Could you check a few things on this drawing? It's one solid part, dimensions in mm from its lowest x, y, z. Round coordinates to 2 decimals unless told otherwise and drop trailing zeros. Write each loop counter-clockwise with the first axis right and the second up, starting at its lowest first coordinate (ties: lowest second). Pieces come first, ordered by that corner, then holes. Notation, with made-up numbers: (51, 52.25) - (71, 52.25) arc R16 ccw to (71, 56.25) - close; hole circle Ø5 at (86, 10). An arc over 180 degrees is marked (long way). Put each result on its own line as item: value.
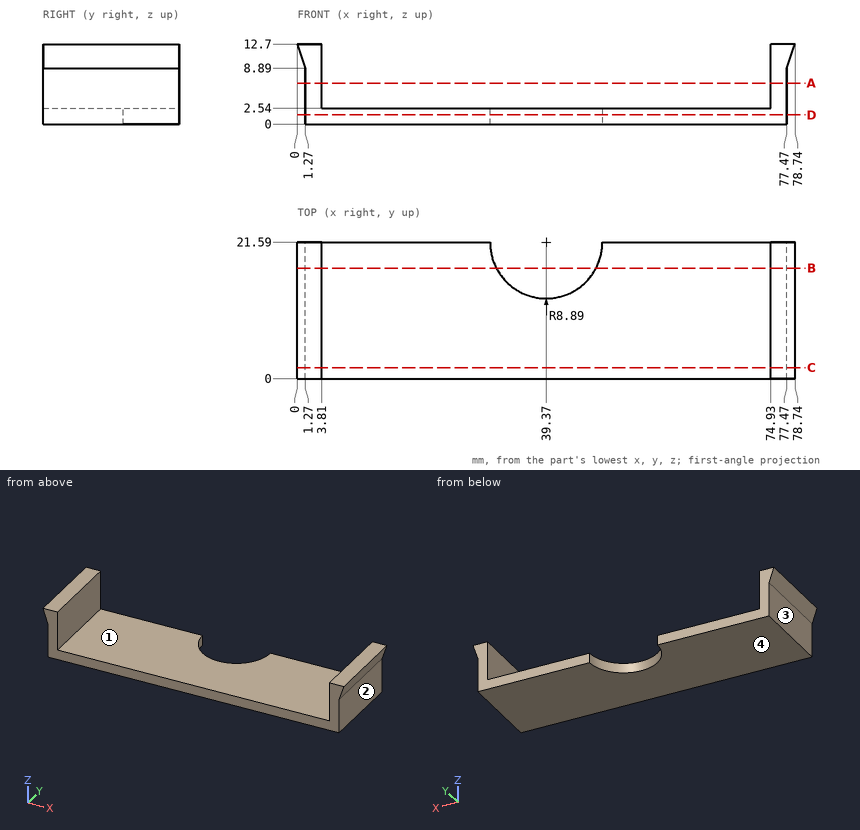
(1) Please list where these lines run through material, in increasing order: probe 1 along X at (y, z) = (20.5, 4.75); probe 2 along Z at (x, y) = (43, 10.5); probe 3 along X at (y, z) = (1, 1). Write a range as from..to.
Values found:
probe 1: x = 1.27..3.81, 74.93..77.47
probe 2: z = 0..2.54
probe 3: x = 1.27..77.47
(2) Imagine slicing it at D-D, the plane z = 1.5. List the corners of the cut face in (x, y) for me.
Values found:
outline: (1.27, 0) - (77.47, 0) - (77.47, 21.59) - (48.26, 21.59) arc R8.89 cw to (30.48, 21.59) - (1.27, 21.59) - close
(3) Imagine slicing it at C-C, the plane y = 1.75. List the corners of the cut face in (x, z) for me, then the cut area to 3 significant figures.
Values found:
outline: (0, 12.7) - (1.27, 8.89) - (1.27, 0) - (77.47, 0) - (77.47, 8.89) - (78.74, 12.7) - (74.93, 12.7) - (74.93, 2.54) - (3.81, 2.54) - (3.81, 12.7) - close
area: 250 mm^2
(4) If we mould it in two halves opening along X, with no side actions, what happens to the marked faces 1, 2, 3 and 4? For each: pulls with the +X half, pulls with the -X half, needs draft (parallel to the pull), parting line crosses it, or undercut.
Values found:
face 1: undercut
face 2: pulls with the +X half
face 3: pulls with the -X half
face 4: needs draft
(5) Imagine slicing it at B-B, the plane y = 17.5. List the corners of the cut face in (x, z) for me, then the cut area to 3 significant figures.
Values found:
outline: (0, 12.7) - (1.27, 8.89) - (1.27, 0) - (31.48, 0) - (31.48, 2.54) - (3.81, 2.54) - (3.81, 12.7) - close; (47.26, 0) - (77.47, 0) - (77.47, 8.89) - (78.74, 12.7) - (74.93, 12.7) - (74.93, 2.54) - (47.26, 2.54) - close
area: 210 mm^2
(6) Imagine slicing it at A-A, the plane z = 6.5. List the corners of the cut face in (x, y) for me, then the cut area to 3 significant figures.
Values found:
outline: (1.27, 0) - (3.81, 0) - (3.81, 21.59) - (1.27, 21.59) - close; (74.93, 0) - (77.47, 0) - (77.47, 21.59) - (74.93, 21.59) - close
area: 110 mm^2
(7) I'm going to push flat-ended pins straight in: pin 1 (3 mm diameter, centred on y = 7.5, z = 8.5, fed in from -X); pin 2 (4 mm diameter, centred on x = 42, y = 4, fed in from +Z); pin 3 (2.5 mm diameter, centred on y = 6.5, z = 5, fed in from +X); pin 4 (3 mm diameter, centred on x = 50.5, y = 18, fed in from -Z). Where does each tip first touch, or does it pass through?
Values found:
pin 1: stops at x = 0.9
pin 2: stops at z = 2.54
pin 3: stops at x = 77.47
pin 4: stops at z = 0
